The listing builds one solid part. Answer for the finished solid, in the listing's coordinates (mm). A direction names the side the tool comes from. Round coordinates to 2 decimals unless told otherwise and drop trailing zeros. Order: outer loops, then holes, each group sorted by start corner. A loop starts at its lowest first (then second) coordinate and runs counter-clockwise, first axis right, second up. Notation, with made-up numbers: (75.5, -17) - (132.5, -17) arc R30 cw to (132.5, 22) - close; hole circle Ø8 at (48, -8). An arc over 180 degrees is marked (long way). Write item = value, one per line.
from build123d import *

# Parameters (mm, degrees)
BOSS_EXTRUDE1_DEPTH = 12.7
CUT_EXTRUDE1_REACH  = 108.324
SKETCH2_R           = 3.175
SKETCH3_R           = 3.175
CUT_EXTRUDE2_DEPTH  = 12.7


with BuildPart() as part:
    # Sketch1 → Boss-Extrude1 (new body)
    with BuildSketch(Plane(origin=(0, 0, 0), x_dir=(1, 0, 0), z_dir=(0, 1, 0))):
        Polygon((0, 0), (-84.328, 0), (-84.328, 63.5), (-71.628, 63.5), (-71.628, 12.7), (-12.7, 12.7), (-12.7, 63.5), (0, 63.5), align=None)
    extrude(amount=BOSS_EXTRUDE1_DEPTH)

    # Cut-Extrude1: up to this face of the body (flat: up to its plane)
    cut_extrude1_end = Plane(part.part.faces().sort_by_distance((-84.328, 6.35, -31.75))[0])
    # Sketch2 → Cut-Extrude1 (cut, up to the picked face)
    with BuildSketch(Plane(origin=(0, 0, 0), x_dir=(0, 0, -1), z_dir=(1, 0, 0)), mode=Mode.PRIVATE) as cut_extrude1_sk1:
        with Locations(Location((57.15, 6.35, 0), (0, 0, 180))):
            Circle(SKETCH2_R)
    cut_extrude1_tool1 = split(extrude(cut_extrude1_sk1.sketch, amount=-CUT_EXTRUDE1_REACH, mode=Mode.PRIVATE), bisect_by=cut_extrude1_end, keep=Keep.BOTH, mode=Mode.PRIVATE)
    add(cut_extrude1_tool1.solids().sort_by(Axis((0, 6.35, -57.15), (-1, 0, 0)))[0], mode=Mode.SUBTRACT)

    # Sketch3 → Cut-Extrude2 (cut)
    with BuildSketch(Plane(origin=(0, 0, -12.7), x_dir=(-1, 0, 0), z_dir=(0, 0, -1))):
        with Locations((45.339, 6.35)):
            Circle(SKETCH3_R)
    extrude(amount=-CUT_EXTRUDE2_DEPTH, mode=Mode.SUBTRACT)


solid = part.part
Q1. Flat-ended cylindrical pins translate along their axes: P1, Ø6.5, axis at y = 8.5, z = -28.5, coming from the +X side; P2, Ø4, axis at x = -34.5, y = 5, coming from the -Z side. Find the tip coordinate at first contact, or state that the pin passes through.
Model answer:
P1 = 0
P2 = -12.7
Q2. Determine the mould class of faces 1 (the face through (-84.328, 6, -31)), 2 (the face through (-42, 0, -11)), 3 (the face through (-42, 12.7, -11)), 4 (the face through (-77.89, 7.57, -54.22)) for opening direction Y: released by +Y, released by -Y, zero draft, split by the parting line, or undercut.
Model answer:
face_1 = zero draft
face_2 = released by -Y
face_3 = released by +Y
face_4 = undercut
Q3. Section D-D on y = 2 is taken. Determine the outline of the cut face in (x, z), then the cut area to 3 significant figures.
Model answer:
outline = (-84.33, -63.5) - (-71.63, -63.5) - (-71.63, -12.7) - (-12.7, -12.7) - (-12.7, -63.5) - (0, -63.5) - (0, 0) - (-84.33, 0) - close
area = 2,360 mm^2
Q4. Find the intervals of material crossed by line 1 (Y direction, x = -76.5, z = -57.15) (3 decimals); line 2 (X direction, y = 11, z = -30); line 3 (Z direction, x = -3.25, y = 6.35) (3 decimals), in increasing order. Write a range as from..to.
Model answer:
line_1 = 0..3.175, 9.525..12.7
line_2 = -84.33..-71.63, -12.7..0
line_3 = -63.5..-60.325, -53.975..0
Q5. Section B-B on z = -31 is taken. Determine the outline of the cut face in (x, y).
Model answer:
outline = (-84.33, 0) - (-71.63, 0) - (-71.63, 12.7) - (-84.33, 12.7) - close; (-12.7, 0) - (0, 0) - (0, 12.7) - (-12.7, 12.7) - close
Q6. Section A-A on y = 6.35 is taken. Determine the outline of the cut face in (x, z) (3 decimals).
Model answer:
outline = (-84.328, -63.5) - (-71.628, -63.5) - (-71.628, -60.325) - (-84.328, -60.325) - close; (-84.328, -53.975) - (-71.628, -53.975) - (-71.628, -12.7) - (-48.514, -12.7) - (-48.514, 0) - (-84.328, 0) - close; (-42.164, -12.7) - (-12.7, -12.7) - (-12.7, -53.975) - (0, -53.975) - (0, 0) - (-42.164, 0) - close; (-12.7, -63.5) - (0, -63.5) - (0, -60.325) - (-12.7, -60.325) - close
Q7. Section C-C on z = -57.15 is taken. Determine the outline of the cut face in (x, y) (3 decimals), then the cut area to 3 significant figures.
Model answer:
outline = (-84.328, 0) - (-71.628, 0) - (-71.628, 3.175) - (-84.328, 3.175) - close; (-84.328, 9.525) - (-71.628, 9.525) - (-71.628, 12.7) - (-84.328, 12.7) - close; (-12.7, 0) - (0, 0) - (0, 3.175) - (-12.7, 3.175) - close; (-12.7, 9.525) - (0, 9.525) - (0, 12.7) - (-12.7, 12.7) - close
area = 161 mm^2
Q8. For faces 5 (the face through (-12.7, 6, -38)), 6 (the face through (0, 6, -32)), determine the directions among +Z, -Z, +X, -X, +Y, -Y from which every point of the face is accessible in a straight line to the end or side of a thin tool.
Model answer:
face_5 = -Z, +Y, -Y
face_6 = +Z, -Z, +X, +Y, -Y
